Part model, mm, in its own coordinate system. Face numbers are marked on the shaded views. Round coordinates to 2 decimals unless told otherwise and drop trailing zeros. Order: outer loops, then holes, each group sorted by start corner. A loop starts at its lowest first (then second) coordinate and runs counter-clockwise, first axis right, second up. Notation, with made-up numbers: (84, 21.25) -> (143, 21.25) arc R13 cw to (143, 31.25) -> close; hole circle Ø3 at (68, 42.25). An arc over 180 degrees is marked (long way). Use CSV: the item, a comma, the result in double quotes.
```python
from build123d import *
from OCP.BRepFilletAPI import BRepFilletAPI_MakeChamfer

# Parameters (mm, degrees)
SKETCH2_W           = 55
SKETCH2_H           = 30
BOSS_EXTRUDE1_DEPTH = 11
CHAMFER1_SIZE       = 10
CHAMFER1_SIZE2      = 8.5
CUT_EXTRUDE1_REACH  = 65.608
SKETCH3_R           = 2.3
SKETCH4_W           = 22
SKETCH4_H           = 7.8
BOSS_EXTRUDE2_DEPTH = 3


with BuildPart() as part:
    # Sketch2 → Boss-Extrude1 (new body)
    with BuildSketch(Plane(origin=(0, 0, 0), x_dir=(1, 0, 0), z_dir=(0, 1, 0))):
        with Locations((27.5, 15)):
            Rectangle(SKETCH2_W, SKETCH2_H)
    extrude(amount=BOSS_EXTRUDE1_DEPTH)

    # Chamfer1: one chamfer whose edges measure the first distance from different faces: ONE call of the kernel's chamfer builder (chamfer() names one face for all edges)
    chamfer1_edges_1 = [part.edges().sort_by_distance(p)[0] for p in [
        (27.5, 11, -30),
    ]]
    chamfer1_side_1 = [part.faces().sort_by_distance(p)[0] for p in [
        (27.5, 5.5, -30),
    ]]
    chamfer1_edges_2 = [part.edges().sort_by_distance(p)[0] for p in [
        (27.5, 11, 0),
    ]]
    chamfer1_side_2 = [part.faces().sort_by_distance(p)[0] for p in [
        (27.5, 5.5, 0),
    ]]
    chamfer1 = BRepFilletAPI_MakeChamfer(part.part.solid().wrapped)
    for e in chamfer1_edges_1:
        chamfer1.Add(CHAMFER1_SIZE, CHAMFER1_SIZE2, e.wrapped, chamfer1_side_1[0].wrapped)  # the first distance lies on this face
    for e in chamfer1_edges_2:
        chamfer1.Add(CHAMFER1_SIZE, CHAMFER1_SIZE2, e.wrapped, chamfer1_side_2[0].wrapped)  # the first distance lies on this face
    add(Compound.cast(chamfer1.Shape()), mode=Mode.REPLACE)

    # Sketch3 → Cut-Extrude1 (cut, up to next)
    with BuildSketch(Plane(origin=(0, 11, 0), x_dir=(1, 0, 0), z_dir=(0, 1, 0)), mode=Mode.PRIVATE) as cut_extrude1_sk1:
        with Locations(Location((6.5, 15, 0), (0, 0, 270))):
            Circle(SKETCH3_R)
    cut_extrude1_tool1 = extrude(cut_extrude1_sk1.sketch, amount=-CUT_EXTRUDE1_REACH, mode=Mode.PRIVATE) & part.part
    # Sketch3 → Cut-Extrude1 (cut, up to next)
    with BuildSketch(Plane(origin=(0, 11, 0), x_dir=(1, 0, 0), z_dir=(0, 1, 0)), mode=Mode.PRIVATE) as cut_extrude1_sk2:
        with Locations(Location((48.5, 15, 0), (0, 0, 270))):
            Circle(SKETCH3_R)
    cut_extrude1_tool2 = extrude(cut_extrude1_sk2.sketch, amount=-CUT_EXTRUDE1_REACH, mode=Mode.PRIVATE) & part.part
    add(cut_extrude1_tool1.solids().sort_by_distance((6.5, 11, -15))[0], mode=Mode.SUBTRACT)
    add(cut_extrude1_tool2.solids().sort_by_distance((48.5, 11, -15))[0], mode=Mode.SUBTRACT)

    # Sketch4 → Boss-Extrude2 (add)
    with BuildSketch(Plane.XZ):
        with Locations((27.5, -14.15)):
            Rectangle(SKETCH4_W, SKETCH4_H)
    extrude(amount=BOSS_EXTRUDE2_DEPTH)


solid = part.part
```
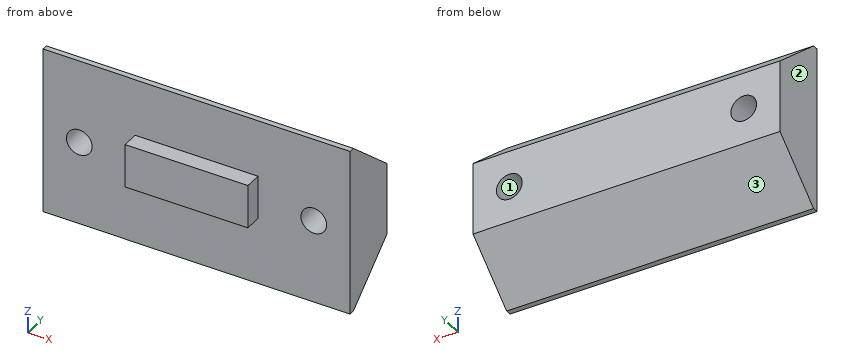
(1) Cut at A-A, the plane x = 6.5. Give the cut face in (y, z), then the cut area to 3 significant figures.
Reply:
outline,"(0, -30) -> (1, -30) -> (11, -21.5) -> (11, -17.3) -> (0, -17.3) -> close; (0, -12.7) -> (11, -12.7) -> (11, -8.5) -> (1, 0) -> (0, 0) -> close"
area,"194 mm2"
(2) Cut at D-D, the plane x = 36. Give the cut face in (y, z).
Reply:
outline,"(-3, -18.05) -> (0, -18.05) -> (0, -30) -> (1, -30) -> (11, -21.5) -> (11, -8.5) -> (1, 0) -> (0, 0) -> (0, -10.25) -> (-3, -10.25) -> close"
(3) Pull direction Z, two halves, no side cores. Call the marked faces 1, 2 and 3: released by +Z, released by -Z, zero draft, split by the parting line, or undercut.
Reply:
face 1,"undercut"
face 2,"zero draft"
face 3,"released by -Z"
(4) Cut at B-B, the plane z = -15. Give the cut face in (x, y).
Reply:
outline,"(0, 0) -> (4.2, 0) -> (4.2, 11) -> (0, 11) -> close; (8.8, 0) -> (16.5, 0) -> (16.5, -3) -> (38.5, -3) -> (38.5, 0) -> (46.2, 0) -> (46.2, 11) -> (8.8, 11) -> close; (50.8, 0) -> (55, 0) -> (55, 11) -> (50.8, 11) -> close"
(5) Drop flat-ended pins along their axis: P1, Ø0.9, axis at x = 23.5, y = -1, coming from the +Z side; P2, Ø2.5, axis at y = -1.5, z = -13.5, coming from the -X side; P3, Ø5, axis at x = 6, z = -11.5, coming from the -Y side. Give the stop position or say it passes through.
Reply:
P1,"z = -10.25"
P2,"x = 16.5"
P3,"y = 0"
(6) Cut at C-C, the plane y = 4. Give the cut face in (x, z), then the cut area to 3 significant figures.
Reply:
outline,"(0, -27.45) -> (55, -27.45) -> (55, -2.55) -> (0, -2.55) -> close; hole circle Ø4.6 at (6.5, -15); hole circle Ø4.6 at (48.5, -15)"
area,"1,340 mm2"
(7) Probe probe 1 along X at (y, z) = (8.5, -15); probe 2 along Y at (x, z) = (47.5, -18.5); probe 3 along X at (y, z) = (2.75, -15.5) (3 decimals). List the from-to ranges inside material, lowest first. Write a range as [from, to].
Reply:
probe 1,"[0, 4.2], [8.8, 46.2], [50.8, 55]"
probe 2,"[0, 11]"
probe 3,"[0, 4.255], [8.745, 46.255], [50.745, 55]"
